Source: CAD feature listing. Evaluate the final solid. Frame: model axes, mm. Face numbers are marked on the shaded views. A direction names the side the tool comes from. Give positions to 0.01 mm unless a question says otherwise; leave off trailing zeros. Order: outer loops, then holes, each group sorted by start corner. A loop starts at its lowest first (then second) coordinate and runs counter-clockwise, first axis right, second up. Notation, with made-up numbers: M -13,65 L 19,65 A25 ccw 19,95 Z; hole C 7.25,34.25 d10. An arc over 180 degrees is marked long. Answer in a Markdown table with one row per item. Add a question column.
(1) Section query D-D, the plane x = 6. Return loops of the section in (y, z), plus the area to 3 significant figures.
(2) Pin query (flat end, axial travel): P1, Ø2, axis at x = 0, z = -1, coming from the -Y side; P2, Ø3, axis at x = 6, z = 0, coming from the +Y side; P3, Ø5, axis at y = -10.5, z = -1.5, coming from the -X side. Return the tip coordinate at first contact, or that it passes through.
(3) Material intervals for line 1 along Y through (x, z) = (1, -5.5); line 2 along Z through (x, y) = (4.75, -13.25); line 3 along Z through (x, y) = (6, -19.35), sorted ascending.
(4) Section query B-B, the plane y = -3. Return loops of the section in (x, z).
(5) Section query A-A, the plane x = -1. Return loops of the section in (y, z), plus the area to 3 significant figures.
(6) Set-up query: the marked faces 1 and 2. Return all of +Z, -Z, +X, -X, +Y, -Y with unobstructed straight access to the full face (end or side cutting, diameter ignored); none if empty.
(7) Mould query, pull axis X, two halves, no side actions, for the marked faces 3, 4 and 5. Classes: pulls with the +X half, pulls with the -X half, needs draft (parallel to the pull), parting line crosses it, or undercut.
(8) Section query C-C, the plane z = 2.5. Return loops of the section in (x, y), plus the area to 3 significant figures.
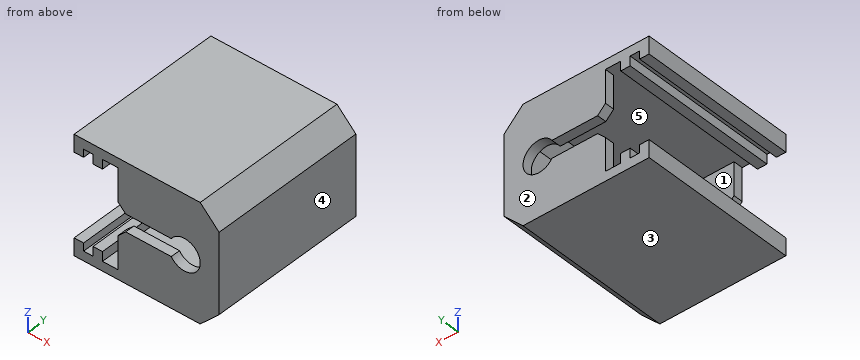
from build123d import *

# Parameters (mm, degrees)
PAD_DEPTH           = 20
PAD001_DEPTH        = 1.2
LINEARPATTERN_COUNT = 2
LINEARPATTERN_PITCH = 18.8


with BuildPart() as part:
    # Sketch → Pad (new body)
    with BuildSketch(Plane.XZ):
        Polygon((-8, 7.45), (8, 7.45), (10.4, 5.05), (10.4, -5.05), (8, -7.45), (-8, -7.45), (-8, -5.25), (-6.8, -5.25), (-6.8, -6.25), (-5.6, -6.25), (-5.6, -5.05), (-4.4, -5.05), (-4.4, -6.25), (7.538299, -6.25), (9.2, -4.588299), (9.2, 4.588299), (7.538299, 6.25), (-4.4, 6.25), (-4.4, 5.05), (-5.6, 5.05), (-5.6, 6.25), (-6.8, 6.25), (-6.8, 5.25), (-8, 5.25), align=None)
    extrude(amount=PAD_DEPTH)

    # Sketch001 (on DatumPlane) → Pad001 (join)
    with BuildSketch(Plane.XZ.offset(20)):
        with BuildLine():
            Line((-2.461701, 6.25), (7.538299, 6.25))
            Line((7.538299, 6.25), (9.2, 4.588299))
            Line((9.2, 4.588299), (9.2, -4.588299))
            Line((9.2, -4.588299), (7.538299, -6.25))
            Line((-2.461701, -6.25), (7.538299, -6.25))
            Line((-2.461701, -6.25), (-2.461701, -2.1))
            Line((-2.461701, -2.1), (-1.461701, -1.1))
            Line((4.329671, -1.1), (-1.461701, -1.1))
            ThreePointArc((4.329671, -1.1), (8, 0), (4.329671, 1.1))
            Line((-1.461701, 1.1), (4.329671, 1.1))
            Line((-1.461701, 1.1), (-2.461701, 2.1))
            Line((-2.461701, 2.1), (-2.461701, 6.25))
        make_face()
    pad001 = extrude(amount=-PAD001_DEPTH)

    # LinearPattern: Pad001 ×2
    with Locations(*[(0, i * LINEARPATTERN_PITCH, 0) for i in range(1, LINEARPATTERN_COUNT)]):
        add(pad001)


solid = part.part
Values follow:
| question | item | result |
|---|---|---|
| 1 | outline | M -20,-7.45 L 0,-7.45 L 0,-2 L -1.2,-2 L -1.2,-6.25 L -18.8,-6.25 L -18.8,-2 L -20,-2 Z; M -20,2 L -18.8,2 L -18.8,6.25 L -1.2,6.25 L -1.2,2 L 0,2 L 0,7.45 L -20,7.45 Z |
| 1 | area | 68.4 mm² |
| 2 | P1 | stops at y = -20 |
| 2 | P2 | passes through |
| 2 | P3 | stops at x = 9.2 |
| 3 | line 1 | y = -20 to -18.8, -1.2 to 0 |
| 3 | line 2 | z = -7.45 to -6.25, 6.25 to 7.45 |
| 3 | line 3 | z = -7.45 to -2, 2 to 7.45 |
| 4 | outline | M -8,-7.45 L 8,-7.45 L 10.4,-5.05 L 10.4,5.05 L 8,7.45 L -8,7.45 L -8,5.25 L -6.8,5.25 L -6.8,6.25 L -5.6,6.25 L -5.6,5.05 L -4.4,5.05 L -4.4,6.25 L 7.54,6.25 L 9.2,4.59 L 9.2,-4.59 L 7.54,-6.25 L -4.4,-6.25 L -4.4,-5.05 L -5.6,-5.05 L -5.6,-6.25 L -6.8,-6.25 L -6.8,-5.25 L -8,-5.25 Z |
| 5 | outline | M -20,-7.45 L 0,-7.45 L 0,-1.1 L -1.2,-1.1 L -1.2,-6.25 L -18.8,-6.25 L -18.8,-1.1 L -20,-1.1 Z; M -20,1.1 L -18.8,1.1 L -18.8,6.25 L -1.2,6.25 L -1.2,1.1 L 0,1.1 L 0,7.45 L -20,7.45 Z |
| 5 | area | 72.7 mm² |
| 6 | face 1 | none |
| 6 | face 2 | +Z, -Z, +X, -X, +Y |
| 7 | face 3 | needs draft |
| 7 | face 4 | pulls with the +X half |
| 7 | face 5 | undercut |
| 8 | outline | M -2.46,-20 L 10.4,-20 L 10.4,0 L -2.46,0 L -2.46,-1.2 L 9.2,-1.2 L 9.2,-18.8 L -2.46,-18.8 Z |
| 8 | area | 52.0 mm² |
